```python
from build123d import *

# Parameters (mm, degrees)
SKETCH1_R               = 4
BOSS_EXTRUDE1_DEPTH     = 3
CROQUIS1_W              = 29
CROQUIS1_H              = 43
SALIENTE_EXTRUIR1_DEPTH = 3
CROQUIS2_R              = 4.25
CORTAR_EXTRUIR1_DEPTH   = 3
CROQUIS4_W              = 3.35
CROQUIS4_H              = 129.34
CORTAR_EXTRUIR2_DEPTH   = 3
CROQUIS5_R              = 4.5
SALIENTE_EXTRUIR2_DEPTH = 3
CROQUIS6_R              = 4.25
CORTAR_EXTRUIR3_DEPTH   = 3


with BuildPart() as part:
    # Sketch1 → Boss-Extrude1 (new body)
    with BuildSketch(Plane.XY):
        Polygon((0, 0), (402.7, 0), (402.7, 86.34), (373.7, 86.34), (373.7, 129.34), (29, 129.34), (29, 86.34), (0, 86.34), align=None)
        with Locations((21.35, 71.34)):
            Circle(SKETCH1_R, mode=Mode.SUBTRACT)
        with Locations((21.35, 15)):
            Circle(SKETCH1_R, mode=Mode.SUBTRACT)
        with Locations((381.35, 15)):
            Circle(SKETCH1_R, mode=Mode.SUBTRACT)
        with Locations((381.35, 71.34)):
            Circle(SKETCH1_R, mode=Mode.SUBTRACT)
        with Locations((199, 15)):
            Circle(SKETCH1_R, mode=Mode.SUBTRACT)
    extrude(amount=BOSS_EXTRUDE1_DEPTH)

    # Croquis1 → Saliente-Extruir1 (add)
    with BuildSketch(Plane.XY.offset(3)):
        with Locations((14.5, 107.84)):
            Rectangle(CROQUIS1_W, CROQUIS1_H)
        with Locations((388.2, 107.84)):
            Rectangle(CROQUIS1_W, CROQUIS1_H)
    extrude(amount=-SALIENTE_EXTRUIR1_DEPTH)

    # Croquis2 → Cortar-Extruir1 (cut)
    with BuildSketch(Plane.XY.offset(3)):
        with Locations((15, 107.84)):
            Circle(CROQUIS2_R)
        with Locations((387.7, 107.84)):
            Circle(CROQUIS2_R)
    extrude(amount=-CORTAR_EXTRUIR1_DEPTH, mode=Mode.SUBTRACT)

    # Croquis4 → Cortar-Extruir2 (cut)
    with BuildSketch(Plane.XY.offset(3)):
        with Locations((1.675, 64.67)):
            Rectangle(CROQUIS4_W, CROQUIS4_H)
        with Locations((401.025, 64.67)):
            Rectangle(CROQUIS4_W, CROQUIS4_H)
    extrude(amount=-CORTAR_EXTRUIR2_DEPTH, mode=Mode.SUBTRACT)

    # Croquis5 → Saliente-Extruir2 (add)
    with BuildSketch(Plane.XY.offset(3)):
        with Locations((199, 15)):
            Circle(CROQUIS5_R)
        with Locations((21.35, 15)):
            Circle(CROQUIS5_R)
        with Locations((21.35, 71.34)):
            Circle(CROQUIS5_R)
        with Locations((15, 107.84)):
            Circle(CROQUIS5_R)
        with Locations((387.7, 107.84)):
            Circle(CROQUIS5_R)
        with Locations((381.35, 71.34)):
            Circle(CROQUIS5_R)
        with Locations((381.35, 15)):
            Circle(CROQUIS5_R)
    extrude(amount=-SALIENTE_EXTRUIR2_DEPTH)

    # Croquis6 → Cortar-Extruir3 (cut)
    with BuildSketch(Plane.XY.offset(3)):
        with Locations((21.35, 107.84)):
            Circle(CROQUIS6_R)
        with Locations((21.35, 15)):
            Circle(CROQUIS6_R)
        with Locations((201.35, 15)):
            Circle(CROQUIS6_R)
        with Locations((381.35, 15)):
            Circle(CROQUIS6_R)
        with Locations((381.35, 107.84)):
            Circle(CROQUIS6_R)
    extrude(amount=-CORTAR_EXTRUIR3_DEPTH, mode=Mode.SUBTRACT)


solid = part.part
```
The listing builds one solid part. Answer for the finished solid, in the listing's coordinates (mm). Give positions to 0.01 mm unless a question says otherwise; leave off trailing zeros. Order: outer loops, then holes, each group sorted by start corner. A loop starts at its lowest first (then second) coordinate and runs counter-clockwise, first axis right, second up.
1) Determine the mould class of faces 1 (the face through (385.276, 106.212, 1.521)), 2 (the face through (199, 66, 0)), 3 (the face through (20.43, 103.69, 1.52)) for opening direction X: pulls with the +X half, pulls with the -X half, needs draft (parallel to the pull), parting line crosses it, or undercut.
Reported:
face 1: undercut
face 2: needs draft
face 3: undercut
2) Find section D-D on x = 201. Write down the section's boundary in (y, z), then the cut area to 3 significant figures.
Reported:
outline: (0, 0) - (10.76, 0) - (10.76, 3) - (0, 3) - close; (19.24, 0) - (129.34, 0) - (129.34, 3) - (19.24, 3) - close
area: 363 mm2
3) Find section A-A on x = 21.35. Write down the section's boundary in (y, z).
Reported:
outline: (0, 0) - (10.75, 0) - (10.75, 3) - (0, 3) - close; (19.25, 0) - (103.59, 0) - (103.59, 3) - (19.25, 3) - close; (112.09, 0) - (129.34, 0) - (129.34, 3) - (112.09, 3) - close
4) Consider line 1 along X through (y, z) = (108.5, 1.55); line 2 along Y through (x, z) = (381.35, 1.7). Determine where each line is inside the solid, lowest interval first.
Reported:
line 1: x = 3.35 to 17.15, 25.55 to 377.15, 385.55 to 399.35
line 2: y = 0 to 10.75, 19.25 to 103.59, 112.09 to 129.34
5) Find section B-B on y = 15. Write down the section's boundary in (x, z), then the cut area to 3 significant figures.
Reported:
outline: (3.35, 0) - (17.1, 0) - (17.1, 3) - (3.35, 3) - close; (25.6, 0) - (197.1, 0) - (197.1, 3) - (25.6, 3) - close; (205.6, 0) - (377.1, 0) - (377.1, 3) - (205.6, 3) - close; (385.6, 0) - (399.35, 0) - (399.35, 3) - (385.6, 3) - close
area: 1,110 mm2
6) Find section C-C on y = 107.84. Write down the section's boundary in (x, z).
Reported:
outline: (3.35, 0) - (17.1, 0) - (17.1, 3) - (3.35, 3) - close; (25.6, 0) - (377.1, 0) - (377.1, 3) - (25.6, 3) - close; (385.6, 0) - (399.35, 0) - (399.35, 3) - (385.6, 3) - close
7) Given P1, Ø10, axis at x = 381.35, y = 15, coming from the -Z side, flat-ended and moving along its own axis, determine where the tip first touches the part or whether it passes through.
Reported:
P1: stops at z = 0
